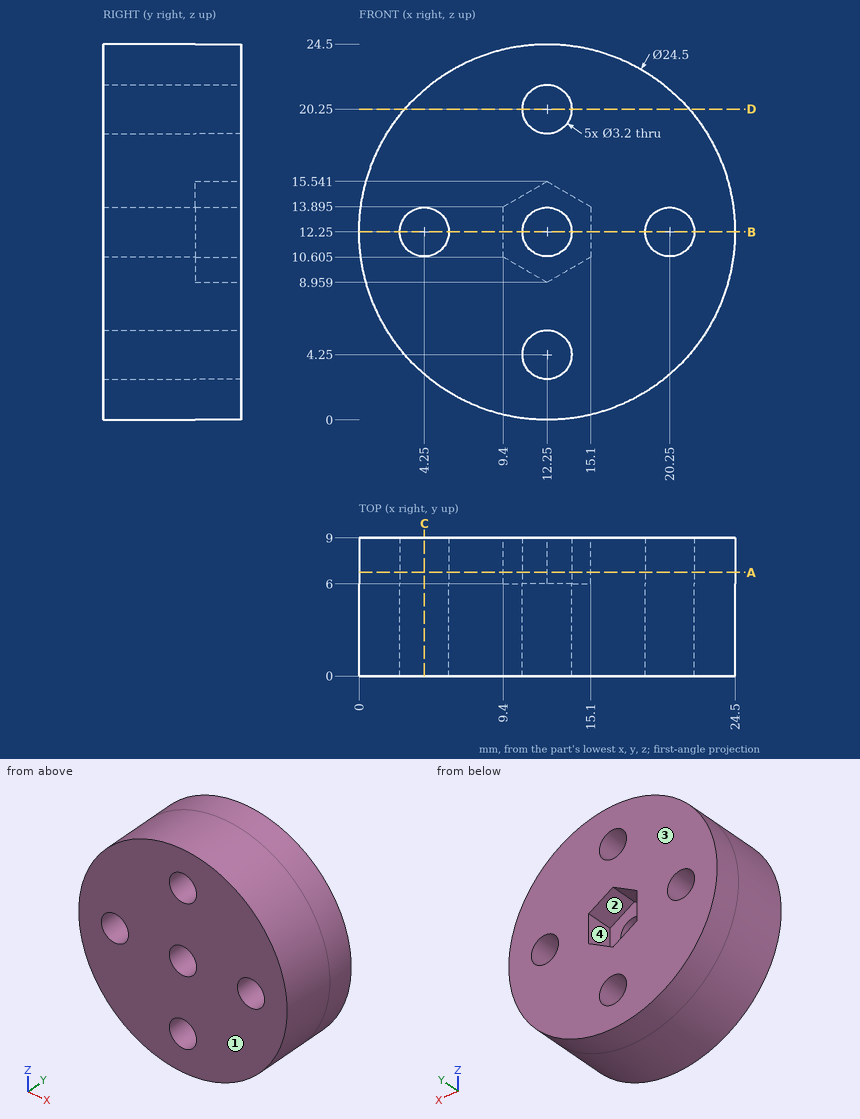
Study the drawing (mm; zero at the part's minimum x, y, z) and answer. A direction names the side the tool comes from. Give positions to 0.01 mm unless a question says otherwise; leave off trailing zeros. Write each loop counter-clockwise with the first axis right and the second up, starting at its lowest first coordinate (ties: lowest second). Pieces come first, ordered by that corner, then holes.
(1) Which of the six approach directions +Z, -Z, +X, -X, +Y, -Y give full straight-line access (tool end or side, diameter ignored) to the marked faces 1 and 2?
Final values:
face 1: +Z, -Z, +X, -X, -Y
face 2: +Y
(2) The part is cut by section A-A on y = 6.75. Count the separate pieces of the cut face and the enclosed holes in it, plus the area to 3 significant figures.
Final values:
separate pieces: 1
enclosed holes: 5
area: 411 mm2
(3) The part is cut by section C-C on x = 4.25. Write down the section's boundary in (y, z).
Final values:
outline: (0, 2.97) - (9, 2.97) - (9, 10.65) - (0, 10.65) - close; (0, 13.85) - (9, 13.85) - (9, 21.53) - (0, 21.53) - close
(4) The mould has two halves that part along X. Classify the marked faces 3 and 4: pulls with the +X half, pulls with the -X half, needs draft (parallel to the pull), parting line crosses it, or undercut.
Final values:
face 3: needs draft
face 4: undercut
(5) Straight lines are drawn through the part: line 1 (Z direction, x = 12, y = 5.75); line 2 (X direction, y = 1.5, z = 13) (1 decimal); line 3 (X direction, y = 2, z = 20.75). For each, find the intervals that lie inside material, in ascending order.
Final values:
line 1: z = 0 to 2.67, 5.83 to 10.67, 13.83 to 18.67, 21.83 to 24.5
line 2: x = 0 to 2.8, 5.7 to 10.8, 13.7 to 18.8, 21.7 to 24.5
line 3: x = 3.43 to 10.73, 13.77 to 21.07
(6) Flat-ended cylindrical pins translate along their axes: pin 1 Ø1.9 at (x, z) = (12.25, 20.25) entering from +Y; pin 2 Ø1 at (x, y) = (18, 4) entering from +Z; pin 3 Ø12 at (x, z) = (17, 18.5) entering from -Y; pin 4 Ø3 at (x, z) = (12.5, 11) entering from +Y. Find the tip coordinate at first contact, or state that the pin passes through.
Final values:
pin 1: passes through
pin 2: stops at z = 23.32
pin 3: stops at y = 0
pin 4: stops at y = 6
(7) The part is cut by section D-D on z = 20.25. Write down the section's boundary in (x, y), plus the area to 3 significant figures.
Final values:
outline: (2.97, 0) - (10.65, 0) - (10.65, 9) - (2.97, 9) - close; (13.85, 0) - (21.53, 0) - (21.53, 9) - (13.85, 9) - close
area: 138 mm2
(8) The part is cut by section B-B on z = 12.25. Write down the section's boundary in (x, y), plus the area to 3 significant figures.
Final values:
outline: (0, 0) - (2.65, 0) - (2.65, 9) - (0, 9) - close; (5.85, 0) - (10.65, 0) - (10.65, 6) - (9.4, 6) - (9.4, 9) - (5.85, 9) - close; (13.85, 0) - (18.65, 0) - (18.65, 9) - (15.1, 9) - (15.1, 6) - (13.85, 6) - close; (21.85, 0) - (24.5, 0) - (24.5, 9) - (21.85, 9) - close
area: 127 mm2
